from build123d import *

# Parameters (mm, degrees)
SKETCH1_W                      = 141
SKETCH1_H                      = 160
BASE_FLANGE3_DEPTH             = 3
EDGE_FLANGE6_STRIP_W           = 13.4732
EDGE_FLANGE6_STRIP_H           = 3
EDGE_FLANGE6_STRIP_CUT_DEPTH   = 160
EDGE_FLANGE6_STRIP_2_W         = 13.4732
EDGE_FLANGE6_STRIP_2_H         = 3
EDGE_FLANGE6_STRIP_CUT_2_DEPTH = 160
EDGE_FLANGE6_DEPTH             = 160
EDGE_FLANGE6_BEND_DEPTH        = 160
EDGE_FLANGE8_STRIP_W           = 13.4732
EDGE_FLANGE8_STRIP_H           = 3
EDGE_FLANGE8_STRIP_CUT_DEPTH   = 160
EDGE_FLANGE8_STRIP_2_W         = 13.4732
EDGE_FLANGE8_STRIP_2_H         = 3
EDGE_FLANGE8_STRIP_CUT_2_DEPTH = 160
EDGE_FLANGE8_DEPTH             = 160
EDGE_FLANGE8_BEND_DEPTH        = 160
SKETCH76_R                     = 4.25
CUT_EXTRUDE1_DEPTH             = 10
CUT_EXTRUDE3_START             = -10
SKETCH80_R                     = 4.25
CUT_EXTRUDE3_DEPTH             = 10
CUT_EXTRUDE4_DEPTH             = 10
SKETCH85_R                     = 4.25
CUT_EXTRUDE5_DEPTH             = 10


# Sheet-metal steps are written as plain solids
with BuildPart() as part:
    # Sketch1 → Base-Flange3 (new body)
    with BuildSketch(Plane(origin=(0, 0, 0), x_dir=(1, 0, 0), z_dir=(0, 1, 0))):
        Rectangle(SKETCH1_W, SKETCH1_H)
    extrude(amount=-BASE_FLANGE3_DEPTH)

    # Edge-Flange6 strip (across the edge) → Edge-Flange6 strip cut (cut)
    with BuildSketch(Plane(origin=(-70.5, -3, 80), x_dir=(1, 0, 0), z_dir=(0, 0, -1))):
        with Locations((-6, -1.5)):
            Rectangle(EDGE_FLANGE6_STRIP_W, EDGE_FLANGE6_STRIP_H)
    extrude(amount=EDGE_FLANGE6_STRIP_CUT_DEPTH, mode=Mode.SUBTRACT)

    # Edge-Flange6 strip 2 (across the edge) → Edge-Flange6 strip cut 2 (cut)
    with BuildSketch(Plane(origin=(70.5, -3, -80), x_dir=(-1, 0, 0), z_dir=(0, 0, 1))):
        with Locations((-6, -1.5)):
            Rectangle(EDGE_FLANGE6_STRIP_2_W, EDGE_FLANGE6_STRIP_2_H)
    extrude(amount=EDGE_FLANGE6_STRIP_CUT_2_DEPTH, mode=Mode.SUBTRACT)

    # Edge-Flange6 section (across the edge) → Edge-Flange6 (add)
    with BuildSketch(Plane(origin=(-70.5, -3, 80), x_dir=(1, 0, 0), z_dir=(0, 0, -1))):
        with BuildLine():
            Line((-3, 0.7366), (-3, 21))
            Line((-3, 21), (0, 21))
            Line((0, 21), (0, 0.7366))
            ThreePointArc((0, 0.7366), (0.215745145, 0.215745145), (0.7366, 0))
            Line((0.7366, 0), (0.7366, -3))
            ThreePointArc((0.7366, -3), (-1.905575199, -1.905575199), (-3, 0.7366))
        make_face()
    extrude(amount=EDGE_FLANGE6_DEPTH)

    # Edge-Flange6 section 2 (across the edge) → Edge-Flange6 bend (add)
    with BuildSketch(Plane(origin=(70.5, -3, -80), x_dir=(-1, 0, 0), z_dir=(0, 0, 1))):
        with BuildLine():
            Line((-3, 0.7366), (-3, 21))
            Line((-3, 21), (0, 21))
            Line((0, 21), (0, 0.7366))
            ThreePointArc((0, 0.7366), (0.215745145, 0.215745145), (0.7366, 0))
            Line((0.7366, 0), (0.7366, -3))
            ThreePointArc((0.7366, -3), (-1.905575199, -1.905575199), (-3, 0.7366))
        make_face()
    extrude(amount=EDGE_FLANGE6_BEND_DEPTH)

    # Edge-Flange8 strip (across the edge) → Edge-Flange8 strip cut (cut)
    with BuildSketch(Plane(origin=(-70.5, -24, 80), x_dir=(0, 1, 0), z_dir=(0, 0, -1))):
        with Locations((-6, -1.5)):
            Rectangle(EDGE_FLANGE8_STRIP_W, EDGE_FLANGE8_STRIP_H)
    extrude(amount=EDGE_FLANGE8_STRIP_CUT_DEPTH, mode=Mode.SUBTRACT)

    # Edge-Flange8 strip 2 (across the edge) → Edge-Flange8 strip cut 2 (cut)
    with BuildSketch(Plane(origin=(70.5, -24, -80), x_dir=(0, 1, 0), z_dir=(0, 0, 1))):
        with Locations((-6, -1.5)):
            Rectangle(EDGE_FLANGE8_STRIP_2_W, EDGE_FLANGE8_STRIP_2_H)
    extrude(amount=EDGE_FLANGE8_STRIP_CUT_2_DEPTH, mode=Mode.SUBTRACT)

    # Edge-Flange8 section (across the edge) → Edge-Flange8 (add)
    with BuildSketch(Plane(origin=(-70.5, -24, 80), x_dir=(0, 1, 0), z_dir=(0, 0, -1))):
        with BuildLine():
            Line((-3, 0.7366), (-3, 12))
            Line((-3, 12), (0, 12))
            Line((0, 12), (0, 0.7366))
            ThreePointArc((0, 0.7366), (0.215745145, 0.215745145), (0.7366, 0))
            Line((0.7366, 0), (0.7366, -3))
            ThreePointArc((0.7366, -3), (-1.905575199, -1.905575199), (-3, 0.7366))
        make_face()
    extrude(amount=EDGE_FLANGE8_DEPTH)

    # Edge-Flange8 section 2 (across the edge) → Edge-Flange8 bend (add)
    with BuildSketch(Plane(origin=(70.5, -24, -80), x_dir=(0, 1, 0), z_dir=(0, 0, 1))):
        with BuildLine():
            Line((-3, 0.7366), (-3, 12))
            Line((-3, 12), (0, 12))
            Line((0, 12), (0, 0.7366))
            ThreePointArc((0, 0.7366), (0.215745145, 0.215745145), (0.7366, 0))
            Line((0.7366, 0), (0.7366, -3))
            ThreePointArc((0.7366, -3), (-1.905575199, -1.905575199), (-3, 0.7366))
        make_face()
    extrude(amount=EDGE_FLANGE8_BEND_DEPTH)

    # Sketch76 → Cut-Extrude1 (cut)
    with BuildSketch(Plane.ZY.offset(73.5)):
        with Locations((-15, -13.5)):
            Circle(SKETCH76_R)
        with BuildLine():
            Line((15, -9.25), (-15, -9.25))
            ThreePointArc((-15, -9.25), (-11.99479618, -10.49479618), (-10.75, -13.5))
            ThreePointArc((-10.75, -13.5), (-11.99479618, -16.50520382), (-15, -17.75))
            Line((-15, -17.75), (15, -17.75))
            ThreePointArc((15, -17.75), (10.75, -13.5), (15, -9.25))
        make_face()
        with Locations((15, -13.5)):
            Circle(SKETCH76_R)
    extrude(amount=-CUT_EXTRUDE1_DEPTH, mode=Mode.SUBTRACT)

    # Sketch80 → Cut-Extrude3 (cut)
    with BuildSketch(Plane(origin=(73.5, 0, 0), x_dir=(0, 0, -1), z_dir=(1, 0, 0)).offset(CUT_EXTRUDE3_START)):
        with Locations((-15, -13.5)):
            Circle(SKETCH80_R)
        with BuildLine():
            Line((15, -9.25), (-15, -9.25))
            ThreePointArc((-15, -9.25), (-11.99479618, -10.49479618), (-10.75, -13.5))
            ThreePointArc((-10.75, -13.5), (-11.99479618, -16.50520382), (-15, -17.75))
            Line((-15, -17.75), (15, -17.75))
            ThreePointArc((15, -17.75), (10.75, -13.5), (15, -9.25))
        make_face()
        with Locations((15, -13.5)):
            Circle(SKETCH80_R)
    extrude(amount=CUT_EXTRUDE3_DEPTH, mode=Mode.SUBTRACT)

    # Sketch84 → Cut-Extrude4 (cut)
    with BuildSketch(Plane(origin=(0, 0, 0), x_dir=(1, 0, 0), z_dir=(0, 1, 0))):
        with BuildLine():
            Line((32.190582692, -56.75), (52.190582692, -56.75))
            ThreePointArc((52.190582692, -56.75), (56.440582692, -52.5), (52.190582692, -48.25))
            Line((52.190582692, -48.25), (32.190582692, -48.25))
            ThreePointArc((32.190582692, -48.25), (27.940582692, -52.5), (32.190582692, -56.75))
        make_face()
        with BuildLine():
            Line((-59.384714022, -56.75), (-39.384714022, -56.75))
            ThreePointArc((-39.384714022, -56.75), (-35.134714022, -52.5), (-39.384714022, -48.25))
            Line((-39.384714022, -48.25), (-59.384714022, -48.25))
            ThreePointArc((-59.384714022, -48.25), (-63.634714022, -52.5), (-59.384714022, -56.75))
        make_face()
        with BuildLine():
            Line((-59.384714022, 48.25), (-39.384714022, 48.25))
            ThreePointArc((-39.384714022, 48.25), (-35.134714022, 52.5), (-39.384714022, 56.75))
            Line((-39.384714022, 56.75), (-59.384714022, 56.75))
            ThreePointArc((-59.384714022, 56.75), (-63.634714022, 52.5), (-59.384714022, 48.25))
        make_face()
        with BuildLine():
            Line((32.190582692, 48.25), (52.190582692, 48.25))
            ThreePointArc((52.190582692, 48.25), (56.440582692, 52.5), (52.190582692, 56.75))
            Line((52.190582692, 56.75), (32.190582692, 56.75))
            ThreePointArc((32.190582692, 56.75), (27.940582692, 52.5), (32.190582692, 48.25))
        make_face()
    extrude(amount=-CUT_EXTRUDE4_DEPTH, mode=Mode.SUBTRACT)

    # Sketch85 → Cut-Extrude5 (cut)
    with BuildSketch(Plane.XZ.offset(3)):
        with Locations(Location((0, 0, 0), (0, 0, 270))):
            Circle(SKETCH85_R)
    extrude(amount=-CUT_EXTRUDE5_DEPTH, mode=Mode.SUBTRACT)


solid = part.part
CAD build for the part. Positions are in the model's coordinates, mm. A direction names the side the tool comes from. Give positions to 0.01 mm unless a question says otherwise; leave off trailing zeros. Write each loop counter-clockwise with the first axis right and the second up, starting at its lowest first coordinate (ties: lowest second). Pieces come first, ordered by that corner, then holes. Notation, with made-up numbers: (-19.75, 61.25) -> (0.25, 61.25) arc R15 cw to (0.25, 81.25) -> close; hole circle Ø3 at (44, -12). An arc over 180 degrees is marked (long way). Return JSON: item names as keys, results as strings.
Item 1: Drop flat-ended pins along their axis: pin 1 (1.5 mm diameter, centred on y = -25, z = 21, fed in from -X); pin 2 (2.5 mm diameter, centred on x = -71.5, z = -6, fed in from +Y); pin 3 (3 mm diameter, centred on x = 26.5, z = 26, fed in from -Y). Give the stop position or say it passes through.
Answer below:
{"pin 1": "stops at x = -73.37", "pin 2": "stops at y = -0.03", "pin 3": "stops at y = -3"}
Item 2: Two-plate mould, pull along X, no slides. Class faces 1 (the cylindrical face through (56.44, -1.48, 52.59)), 2 (the flat face through (64, -27, -1)), 3 (the cylindrical face through (72.38, -1.07, -1.12)), 4 (the cylindrical face through (-72.43, -25.88, 1.12)): +X half, -X half, draft (parallel to the pull), parting line (faces both ways), or undercut.
Answer below:
{"face 1": "undercut", "face 2": "draft", "face 3": "+X half", "face 4": "-X half"}
Item 3: Band-saw the part on A-A (y = -19.75). List the corners of the cut face in (x, z), then the cut area to 3 significant figures.
Answer below:
{"outline": "(-73.5, -80) -> (-70.5, -80) -> (-70.5, 80) -> (-73.5, 80) -> close; (70.5, -80) -> (73.5, -80) -> (73.5, 80) -> (70.5, 80) -> close", "area": "960 mm2"}
Item 4: Band-saw the part on C-C (z = 0). Give the number of separate pieces and of enclosed holes in the cut face, then the cut area to 3 significant figures.
Answer below:
{"separate pieces": "4", "enclosed holes": "0", "area": "569 mm2"}
Item 5: Tool access for faces 5 (the flat face through (15, -3, -1)), 6 (the cylindrical face through (71.98, -13.59, -19.25)), 7 (the cylindrical face through (-63.634, -1.479, -52.593)): list every direction of +Z, -Z, +X, -X, +Y, -Y with a clear straight run to the whole face (end or side of a thin tool).
Answer below:
{"face 5": "+Z, -Z", "face 6": "+X, -X", "face 7": "+Y"}
Item 6: Band-saw the part on B-B (x = 36.5). List the corners of the cut face in (y, z), then the cut area to 3 significant figures.
Answer below:
{"outline": "(-3, -80) -> (0, -80) -> (0, -56.75) -> (-3, -56.75) -> close; (-3, -48.25) -> (0, -48.25) -> (0, 48.25) -> (-3, 48.25) -> close; (-3, 56.75) -> (0, 56.75) -> (0, 80) -> (-3, 80) -> close", "area": "429 mm2"}
Item 7: Drill centre lines: probe 1 along Z at (x, y) = (-41, -2); probe 2 along X at (y, z) = (-21, -37.5); probe 3 along Y at (x, z) = (-67, -47). Where is each one in solid material? Low to high.
Answer below:
{"probe 1": "z = -80 to -56.75, -48.25 to 48.25, 56.75 to 80", "probe 2": "x = -73.5 to -70.5, 70.5 to 73.5", "probe 3": "y = -27 to -24, -3 to 0"}
Item 8: Band-saw the part on D-D (x = 0). List the corners of the cut face in (y, z).
Answer below:
{"outline": "(-3, -80) -> (0, -80) -> (0, -4.25) -> (-3, -4.25) -> close; (-3, 4.25) -> (0, 4.25) -> (0, 80) -> (-3, 80) -> close"}
